Here's how the part is built. I have some questions about the finished solid (model axes, mm). A direction names the side the tool comes from. Give positions to 0.01 mm unless a question says otherwise; leave off trailing zeros. Order: outer loops, then holes, each group sorted by start corner. A loop starts at its lowest first (then second) coordinate and runs counter-clockwise, first axis right, second up. Notation, with made-up numbers: M 52,27 L 86,27 A19 cw 86,50 Z; hole C 64,-28.5 d5. An arc over 180 degrees is marked long. One line per item, written item: value. Start each with the question number.
from build123d import *

# Parameters (mm, degrees)
SKETCH1_R           = 135
BOSS_EXTRUDE1_DEPTH = 700
SKETCH2_W           = 296.361167152
SKETCH2_H           = 281.411070578
BOSS_EXTRUDE2_DEPTH = 20.32
SHELL1_T            = -20.32
SHELL2_START        = -20.32
SHELL2_DEPTH        = 20.32
BOSS_EXTRUDE3_DEPTH = 13.97
BOSS_EXTRUDE4_DEPTH = 13.97
BOSS_EXTRUDE5_DEPTH = 6.604


# Read off the part's stored shape, not the designer's step: Shell2
with BuildPart() as part:
    # Sketch1 → Boss-Extrude1 (new body)
    with BuildSketch(Plane(origin=(0, 0, 0), x_dir=(1, 0, 0), z_dir=(0, 1, 0))):
        with Locations(Location((0, 0, 0), (0, 0, 270))):
            Circle(SKETCH1_R)
    extrude(amount=BOSS_EXTRUDE1_DEPTH)

    # Sketch2 → Boss-Extrude2 (add)
    with BuildSketch(Plane(origin=(0, 0, 0), x_dir=(-1, 0, 0), z_dir=(0, -1, 0))):
        Rectangle(SKETCH2_W, SKETCH2_H)
    extrude(amount=BOSS_EXTRUDE2_DEPTH)

    # Shell1
    shell1_openings = [part.faces().sort_by_distance(p)[0] for p in [
        (0, 700, 0),
    ]]
    offset(amount=SHELL1_T, openings=shell1_openings, kind=Kind.INTERSECTION)

    # Shell2 outline → Shell2 (cut)
    with BuildSketch(Plane(origin=(0, 0, 0), x_dir=(1, 0, 0), z_dir=(0, 1, 0)).offset(SHELL2_START)):
        with BuildLine():
            Line((-127.860583576, -43.320562873), (-127.860583576, -120.385535289))
            Line((-127.860583576, -120.385535289), (-61.092740103, -120.385535289))
            ThreePointArc((-61.092740103, -120.385535289), (-102.032309224, -88.399139557), (-127.860583576, -43.320562873))
        make_face()
        with BuildLine():
            Line((-127.860583576, 120.385535289), (-127.860583576, 43.320562873))
            ThreePointArc((-127.860583576, 43.320562873), (-102.032309224, 88.399139557), (-61.092740103, 120.385535289))
            Line((-61.092740103, 120.385535289), (-127.860583576, 120.385535289))
        make_face()
        with BuildLine():
            ThreePointArc((127.860583576, -43.320562873), (102.032309224, -88.399139557), (61.092740103, -120.385535289))
            Line((61.092740103, -120.385535289), (127.860583576, -120.385535289))
            Line((127.860583576, -120.385535289), (127.860583576, -43.320562873))
        make_face()
        with BuildLine():
            Line((127.860583576, 120.385535289), (61.092740103, 120.385535289))
            ThreePointArc((61.092740103, 120.385535289), (102.032309224, 88.399139557), (127.860583576, 43.320562873))
            Line((127.860583576, 43.320562873), (127.860583576, 120.385535289))
        make_face()
    extrude(amount=SHELL2_DEPTH, mode=Mode.SUBTRACT)

    # Sketch3 → Boss-Extrude3 (add)
    with BuildSketch(Plane.ZY.offset(148.180583576)):
        Polygon((-140.705535289, 0), (142.300478433, 168.1079442), (140.705535289, 0), align=None)
    extrude(amount=-BOSS_EXTRUDE3_DEPTH)

    # Sketch4 → Boss-Extrude4 (add)
    with BuildSketch(Plane(origin=(148.180583576, 0, 0), x_dir=(0, 0, -1), z_dir=(1, 0, 0))):
        Polygon((140.705535289, 0), (-139.866409205, 168.107944167), (-140.705535289, 0), align=None)
    extrude(amount=-BOSS_EXTRUDE4_DEPTH)

    # Sketch6 → Boss-Extrude5 (add)
    with BuildSketch(Plane.XY.offset(140.705535289)):
        Polygon((134.162146303, 168.27987687), (-133.500855759, 168.27987687), (-134.210583576, 0), (134.210583576, 0), align=None)
    extrude(amount=-BOSS_EXTRUDE5_DEPTH)


solid = part.part
Item 1: I want a section at B-B on x = 0. Write out the boundary of the cut face in (y, z).
Item 2: Will these pins go through, and if not, where does the flat tip stop? P1, Ø5, axis at y = 601.5, z = -21.5, coming from the -X side; P2, Ø6, axis at y = 385.5, z = 41.5, coming from the +X side; P3, Ø1.5, axis at x = 66, y = 568.5, coming from the +Z side.
Item 3: For faces 5 (the face through (134.211, 67, 79)), 6 (the face through (34.4, 345.1, 109.4)), 7 (the face through (-148.181, 54, 34)), which set-ups out of +Z, -Z, +X, -X, +Y, -Y let a thin tool reach every point of the face, with its end or its side?
Item 4: I want a section at D-D on z = -86. Write out the boundary of the cut face in (x, y), plus the area to 3 significant figures.
Item 5: Please list where these lines run through material, in increasing order: probe 1 along X at (y, z) = (401, 0); probe 2 along Z at (x, y) = (-54, 78); probe 3 along Y at (x, z) = (51, -60.5). Write a range as [from, to].
Item 6: We'd pull the mould along Z, two halves only. Please class faces 1 (the face through (-2, 75, 140.706)), 2 (the face through (-76, 85, 134.102)), 3 (the face through (1, 0, -139)), 4 (the face through (106, 0, 123)): +Z half, -Z half, draft (parallel to the pull), parting line (faces both ways), or undercut.
Item 7: I want a section at A-A on z = -53.5. Write out the boundary of the cut face in (x, y).
Item 8: I want a section at C-C on y = 196. Write out the boundary of the cut face in (x, z), plus the area to 3 significant figures.
Answer below:
1. outline: M -20.32,-140.71 L 0,-140.71 L 0,-135 L 700,-135 L 700,-114.68 L 0,-114.68 L 0,114.68 L 700,114.68 L 700,135 L 168.28,135 L 168.28,140.71 L -20.32,140.71 Z
2. P1: stops at x = -133.66
2. P2: stops at x = 129.39
2. P3: stops at z = 118.18
3. face 5: none
3. face 6: +Y
3. face 7: +Z, -Z, -X, +Y, -Y
4. outline: M -148.18,-20.32 L -127.86,-20.32 L -127.86,0 L -134.21,0 L -134.21,32.5 L -148.18,32.5 Z; M -104.06,-20.32 L 104.06,-20.32 L 104.06,700 L 75.87,700 L 75.87,0 L -75.87,0 L -75.87,700 L -104.06,700 Z; M 127.86,-20.32 L 148.18,-20.32 L 148.18,32.78 L 134.21,32.78 L 134.21,0 L 127.86,0 Z
4. area: 45,400 mm²
5. probe 1: x = [-135, -114.68], [114.68, 135]
5. probe 2: z = [-123.73, -101.17], [101.17, 123.73], [134.1, 140.71]
5. probe 3: y = [-20.32, 0]
6. face 1: +Z half
6. face 2: undercut
6. face 3: draft
6. face 4: undercut
7. outline: M -148.18,-20.32 L -127.86,-20.32 L -127.86,0 L -134.21,0 L -134.21,51.8 L -148.18,51.8 Z; M -123.95,-20.32 L 123.95,-20.32 L 123.95,700 L 101.44,700 L 101.44,0 L -101.44,0 L -101.44,700 L -123.95,700 Z; M 127.86,-20.32 L 148.18,-20.32 L 148.18,52.25 L 134.21,52.25 L 134.21,0 L 127.86,0 Z
8. outline: C 0,0 d270; hole C 0,0 d229.36
8. area: 15,900 mm²
